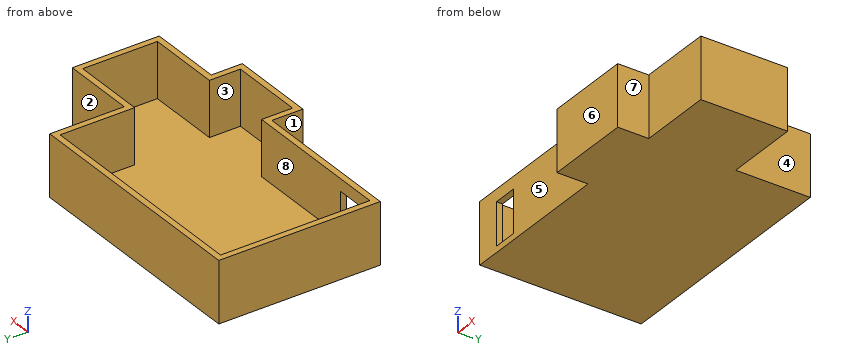
from build123d import *

# Parameters (mm, degrees)
F1_DEPTH = 25
F2_T     = -2.5
F3_W     = 10
F3_H     = 20
F4_DEPTH = 2.5
F5_DEPTH = 2.5


with BuildPart() as f1:
    # F0 (on Top) → F1 (new body)
    with BuildSketch(Plane.XY):
        Polygon((-73.6584961414, 55.3277601087), (-73.6584961414, -10.7122398913), (-10.1584961414, -10.7122398913), (-10.1584961414, -23.4122398913), (25.4015038586, -23.4122398913), (25.4015038586, -10.7122398913), (55.8815038586, -10.7122398913), (55.8815038586, 24.8477601087), (25.4015038586, 24.8477601087), (25.4015038586, 55.3277601087), align=None)
    extrude(amount=F1_DEPTH)

    # F2
    f2_openings = [f1.faces().sort_by_distance(p)[0] for p in [
        (-13.662154, 18.061578, 25),
    ]]
    offset(amount=F2_T, openings=f2_openings, kind=Kind.INTERSECTION)

    # F3 (on face) → F4 (cut)
    with BuildSketch(Plane.XZ.offset(10.7122398913)):
        with Locations((-58.8584271073, 10)):
            Rectangle(F3_W, F3_H)
    extrude(amount=-F4_DEPTH, mode=Mode.SUBTRACT)

    # F5 (add): a face of the model
    f5_faces = [f1.faces().sort_by_distance(p)[0] for p in [
        (-58.8584271073, -8.2122398913, 1.25),
    ]]
    extrude(f5_faces, amount=F5_DEPTH)


solid = f1.part
Read the model definition and answer for the solid it produces. Units are mm, in the model's axes. Face numbers are marked on the shaded views. A direction names the side the tool comes from. Coordinates: 2 decimals unless noted, no trailing zeros. Loops run counter-clockwise (first coordinate to the right, second up) from the corner with the lowest first, then second, coordinate; pieces in that order, holes last.
Q1. The part is cut by section B-B on y = -14. Write down the section's boundary in (x, z).
Q2. The part is cut by section C-C on x = 21. Write down the section's boundary in (y, z).
Q3. Consider probe 1 along Y at (x, z) = (9, 5.5); probe 2 along Y at (x, z) = (37, 6.75); probe 3 along X at (y, z) = (11, 22.75). Determine where each line is inside the solid, lowest interval first.
Q4. The mould has two halves that part along X. Classify the marked faces 1, 2, 3 and 4: +X half, -X half, draft (parallel to the pull), parting line (faces both ways), or undercut.
Q5. Each of these flat-tipped pins is pushed along its axis until it touches: pin 1 Ø5 at (x, z) = (-44.5, 4.5) entering from -Y; pin 2 Ø10 at (y, z) = (-17.5, 13.5) entering from -X; pin 3 Ø12.5 at (y, z) = (39, 16) entering from +X; pin 4 Ø10 at (y, z) = (-14.5, 14.5) entering from +X. Where does it stop, or does it pass through?
Q6. Which of the six approach directions +Z, -Z, +X, -X, +Y, -Y give full straight-line access (tool end or side, diameter ignored) to the marked faces 5, 6, 7 and 8?
Q7. The part is cut by section A-A on z = 5.75. Write down the section's boundary in (x, y), and give its area (3 significant figures).
Results below:
1. outline: (-10.16, 0) - (25.4, 0) - (25.4, 25) - (22.9, 25) - (22.9, 2.5) - (-7.66, 2.5) - (-7.66, 25) - (-10.16, 25) - close
2. outline: (-23.41, 0) - (55.33, 0) - (55.33, 25) - (52.83, 25) - (52.83, 2.5) - (-20.91, 2.5) - (-20.91, 25) - (-23.41, 25) - close
3. probe 1: y = -23.41 to -20.91, 52.83 to 55.33
3. probe 2: y = -10.71 to -8.21, 22.35 to 24.85
3. probe 3: x = -73.66 to -71.16, 53.38 to 55.88
4. face 1: -X half
4. face 2: draft
4. face 3: undercut
4. face 4: +X half
5. pin 1: stops at y = -10.71
5. pin 2: stops at x = -10.16
5. pin 3: stops at x = 25.4
5. pin 4: stops at x = 55.88
6. face 5: +Z, -Z, -X, -Y
6. face 6: +Z, -Z, +X, -X, -Y
6. face 7: +Z, -Z, +X, -Y
6. face 8: +Z
7. outline: (-73.66, -10.71) - (-63.86, -10.71) - (-63.86, -8.21) - (-71.16, -8.21) - (-71.16, 52.83) - (22.9, 52.83) - (22.9, 22.35) - (53.38, 22.35) - (53.38, -8.21) - (22.9, -8.21) - (22.9, -20.91) - (-7.66, -20.91) - (-7.66, -8.21) - (-53.86, -8.21) - (-53.86, -10.71) - (-10.16, -10.71) - (-10.16, -23.41) - (25.4, -23.41) - (25.4, -10.71) - (55.88, -10.71) - (55.88, 24.85) - (25.4, 24.85) - (25.4, 55.33) - (-73.66, 55.33) - close
7. area: 991 mm2
